Autodesk Inventor part; units mm, degrees
ref_plane "Work Plane1" through (36.1864, 42.3186, 5) normal (0.3051918, 0.9522909, 0) x (0.9522909, -0.3051918, 0)
ref_plane "YZ Plane" through (0, 0, 0) normal (1, 0, 0) x (0, 1, 0)
ref_plane "XZ Plane" through (0, 0, 0) normal (0, 1, 0) x (-1, 0, 0)
sketch "Sketch1" plane through (0, 0, 0) normal (0, 0, 1) x (1, 0, 0)
  circle A0 centre (17.6, 46.7) radius 1.2
  circle A1 centre (35.8812, 41.3663) radius 1.3
  arc A2 (18.5156, 49.5569) -> (17.5984, 43.7) centre (17.6, 46.7) ccw
  arc A3 (33.4647, 40.7254) -> (36.6442, 43.747) centre (35.8812, 41.3663) ccw
  line L0 (18.5156, 49.5569) -> (36.6442, 43.747)
  line L1 (17.5984, 43.7) -> (29.5984, 43.7)
  arc A4 (33.4647, 40.7254) -> (29.5984, 43.7) centre (29.5984, 39.7) ccw
  point P0 (0, 0)
  dimension "d0" = 5
  dimension "d1" = 3
  dimension "d3" = 4
  dimension "d14" = 12
extrude "Extrusion1" add sketch "Sketch1" along normal mid plane 10
ref_plane "Work Plane1" through (36.1864, 42.3186, 5) normal (0.3051918, 0.9522909, 0) x (0.9522909, -0.3051918, 0)
sketch "Sketch2" plane through (36.1864, 42.3186, 5) normal (0.3051918, 0.9522909, 0) x (0.9522909, -0.3051918, 0)
  line L0 (8.5468, 5) -> (-28.0353, 5)
  line L1 (-22.0368, 8.5) -> (2.5, 8.5)
  line L2 (2.5, 8.5) -> (2.5, 1.5)
  line L3 (2.5, 1.5) -> (-22.0368, 1.5)
  line L4 (-22.0368, 1.5) -> (-22.0368, 8.5)
  line L5 (2.5, 10) -> (2.5, 0)
  line L6 (-22.0368, 10) -> (-22.0368, 0)
  point P0 (-21.5447, 5)
  dimension "d7" = 7
extrude "Extrusion2" cut sketch "Sketch2" against normal through all
sketch "Sketch3" plane through (36.1864, 42.3186, 5) normal (-0.3051918, -0.9522909, 0) x (0.9522909, -0.3051918, 0)
  line L0 (-21.6349, -8.5) -> (-21.6349, -1.5)
  line L1 (-21.6349, -8.5) -> (2.2913, -8.5)
  line L2 (2.2913, -1.5) -> (2.2913, -8.5)
  line L3 (-21.6349, -1.5) -> (-17.6349, -1.5)
  line L4 (-17.6349, -1.5) -> (-17.6349, -8.5)
  line L5 (-17.6349, -8.5) -> (-21.6349, -8.5)
  line L6 (-21.6349, -8.5) -> (-21.6349, -1.5)
  line L7 (2.2913, -1.5) -> (-1.7087, -1.5)
  line L8 (-1.7087, -1.5) -> (-1.7087, -8.5)
  line L9 (-1.7087, -8.5) -> (2.2913, -8.5)
  line L10 (2.2913, -8.5) -> (2.2913, -1.5)
  point P0 (-21.5447, -5)
  dimension "d10" = 4
  dimension "d11" = 4
extrude "Extrusion3" cut sketch "Sketch3" against normal through all
properties part number "Lever for inset hinge" material "Steel"
Check sheet for the modelled part. Datum: model origin and axes. Units: mm. A direction names the side the tool comes from. Round coordinates to 2 decimals unless told otherwise and drop trailing zeros. Order: outer loops, then holes, each group sorted by start corner. A loop starts at its lowest first (then second) coordinate and runs counter-clockwise, first axis right, second up.
Q1. Set-up check for faces 1 (the face through (34.785, 43.544, 0.049)), 2 (the face through (26.87, 45.304, -0.049)), 3 (the face through (24, 43.7, -4)), 4 (the face through (17.34, 47.87, -4.26)): record each of +Z, -Z, +X, -X, +Y, -Y from which the full face is reachable in a straight line by a thin tool's end or side.
Filled sheet:
face 1: +X, -Y
face 2: -X, -Y
face 3: +Z, -Z, -X, -Y
face 4: +Z, -Z
Q2. Cross-section at B-B, the plane z = -4.5. Enter the section's corners in (x, y).
Filled sheet:
outline: (17.6, 43.7) - (29.6, 43.7) arc R4 cw to (33.46, 40.73) arc R2.5 ccw (long way) to (36.64, 43.75) - (18.52, 49.56) arc R3 ccw (long way) to start; hole circle Ø2.4 at (17.6, 46.7); hole circle Ø2.6 at (35.88, 41.37)
Q3. Scan lines: L1, parallel to Y at x = 17.6, z = -4.5; L2, parallel to Z at x = 34.5, y = 39.75; L3, parallel to Y at x = 28, z = 2. Record each from-to range of solid material in increasing order.
Filled sheet:
L1: y = 43.7 to 45.5, 47.9 to 49.7
L2: z = -5 to -3.5, 3.5 to 5
L3: y = 44.94 to 46.52
Q4. Draft check along Y on faces 5 (the face through (26, 45, -5)), 6 (the face through (17.34, 47.87, 4.24)), 7 (the face through (19.619, 48.405, 0.049)), 8 (the face through (36.48, 42.52, -4.26)). Enter one of: pulls with the +Y half, pulls with the -Y half, needs draft (parallel to the pull), parting line crosses it, or undercut.
Filled sheet:
face 5: needs draft
face 6: undercut
face 7: pulls with the +Y half
face 8: undercut
Q5. Cross-section at A-A, the plane y = 46.7. Enter the section's corners in (x, z).
Filled sheet:
outline: (14.6, -5) - (16.4, -5) - (16.4, -3.5) - (14.6, -3.5) - close; (14.6, 3.5) - (16.4, 3.5) - (16.4, 5) - (14.6, 5) - close; (18.8, -5) - (27.43, -5) - (27.43, 5) - (18.8, 5) - (18.8, 3.5) - (22.52, 3.5) - (22.52, -3.5) - (18.8, -3.5) - close
Q6. Depth check by flat-ended pin: P1, Ø1.6, axis at x = 26.5, z = 4, coming from the -Y side; P2, Ø1.5, axis at x = 31.5, z = -0.5, coming from the -Y side; P3, Ø3, axis at x = 28.5, z = 4, coming from the +Y side. Enter the tip coordinate at first touch or a pass-through.
Filled sheet:
P1: stops at y = 43.7
P2: stops at y = 43.58
P3: stops at y = 46.84
Q7. Cross-section at D-D, the plane y = 48.25. Enter the section's corners in (x, z), plus the area to 3 significant figures.
Filled sheet:
outline: (15.03, -5) - (22.59, -5) - (22.59, 5) - (15.03, 5) - (15.03, 3.5) - (19.57, 3.5) - (19.57, -3.5) - (15.03, -3.5) - close
area: 43.9 mm2
Q8. Cross-section at C-C, the plane x = 34. Enter the section's corners in (y, z), plus the area to 3 significant figures.
Filled sheet:
outline: (39.72, -5) - (44.59, -5) - (44.59, 5) - (39.72, 5) - (39.72, 3.5) - (43.02, 3.5) - (43.02, -3.5) - (39.72, -3.5) - close
area: 25.7 mm2
